Could you check a few things on this drawing? It's one solid part, dimensions in mm from its lowest x, y, z. A direction names the side the tool comes from. Give positions to 0.01 mm unless a question says otherwise; leave off trailing zeros. Write each loop counter-clockwise with the first axis right and the second up, starting at its lowest first coordinate (ties: lowest second). Pieces come first, ordered by that corner, then holes.
1. Suppose I cut it at C-C (x = 24.5). Please give me the cut outline in (y, z).
2. I'm going to push flat-ended pins straight in: pin 1 (4 mm diameter, centred on x = 32, y = 23, fed in from +Z); pin 2 (2 mm diameter, centred on x = 44, y = 60, fed in from -Z); pin 3 (12 mm diameter, centred on x = 7, y = 21, fed in from +Z); pin 4 (4 mm diameter, centred on y = 40.5, z = 19, fed in from -X). Where does each tip first touch, or does it pass through?
3. Suppose I cut it at A-A (z = 7.25). Please give me the cut outline in (x, y), and give its area (3 significant figures).
4. Suppose I cut it at B-B (y = 60). Please give me the cut outline in (x, z), and give its area (3 significant figures).
5. If I drill on probe 1 along X at (y, z) = (38.5, 16.25); probe 2 along Y at (x, z) = (44, 1.95); probe 3 along Y at (x, z) = (56.2, 16), over which ranges is the centre line in solid material (lowest first)?
6. On a 3-axis mill with a long thin cutter (end or side, diameter ignored), from which of +Z, -Z, +X, -X, +Y, -Y can I reach the whole of each face in a straight line? I mean the marked faces 1, 2, 3 and 4. Say none if no direction works.
7. Suppose I cut it at D-D (x = 48). Please give me the cut outline in (y, z), and give its area (4 significant figures).
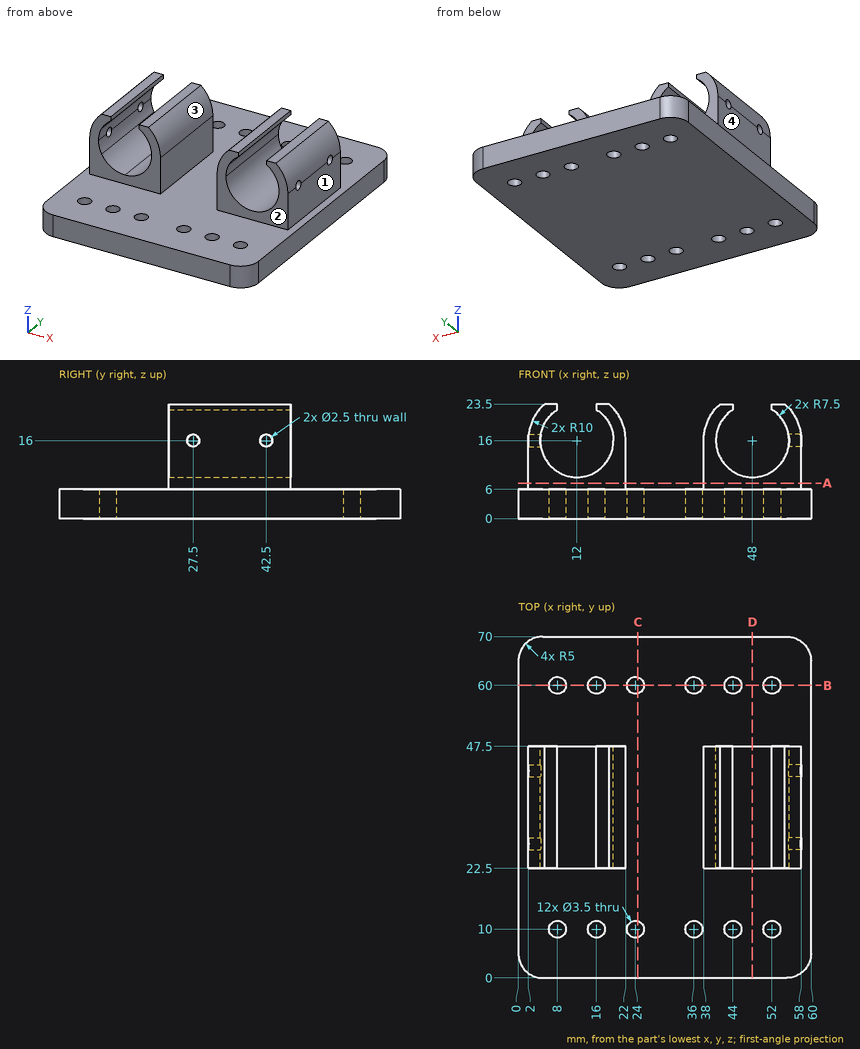
Checks:
1. outline: (0, 0) - (8.32, 0) - (8.32, 6) - (0, 6) - close; (11.68, 0) - (58.32, 0) - (58.32, 6) - (11.68, 6) - close; (61.68, 0) - (70, 0) - (70, 6) - (61.68, 6) - close
2. pin 1: stops at z = 6
2. pin 2: passes through
2. pin 3: stops at z = 23.5
2. pin 4: stops at x = 2.05
3. outline: (2, 22.5) - (22, 22.5) - (22, 47.5) - (2, 47.5) - close; (38, 22.5) - (58, 22.5) - (58, 47.5) - (38, 47.5) - close
3. area: 1,000 mm2
4. outline: (0, 0) - (6.25, 0) - (6.25, 6) - (0, 6) - close; (9.75, 0) - (14.25, 0) - (14.25, 6) - (9.75, 6) - close; (17.75, 0) - (22.25, 0) - (22.25, 6) - (17.75, 6) - close; (25.75, 0) - (34.25, 0) - (34.25, 6) - (25.75, 6) - close; (37.75, 0) - (42.25, 0) - (42.25, 6) - (37.75, 6) - close; (45.75, 0) - (50.25, 0) - (50.25, 6) - (45.75, 6) - close; (53.75, 0) - (60, 0) - (60, 6) - (53.75, 6) - close
4. area: 234 mm2
5. probe 1: x = 2 to 4.5, 19.5 to 22, 38 to 40.5, 55.5 to 58
5. probe 2: y = 0 to 8.25, 11.75 to 58.25, 61.75 to 70
5. probe 3: y = 22.5 to 26.25, 28.75 to 41.25, 43.75 to 47.5
6. face 1: +Z, +X, +Y, -Y
6. face 2: +Z, +X, -X, -Y
6. face 3: +Z, +Y, -Y
6. face 4: +Z, -X, +Y, -Y
7. outline: (0, 0) - (70, 0) - (70, 6) - (47.5, 6) - (47.5, 8.5) - (22.5, 8.5) - (22.5, 6) - (0, 6) - close
7. area: 482.5 mm2
